from build123d import *

# Parameters (mm, degrees)
SKETCH1_R           = 3
BOSS_EXTRUDE1_DEPTH = 1.3
CHAMFER1_SIZE       = 1
SKETCH2_R           = 2
BOSS_EXTRUDE2_DEPTH = 2
CUT_EXTRUDE3_DEPTH  = 1
FILLET1_R           = 0.1
FILLET2_R           = 0.1


with BuildPart() as part:
    # Sketch1 → Boss-Extrude1 (new body)
    with BuildSketch(Plane(origin=(0, 0, 0), x_dir=(0, 0, -1), z_dir=(1, 0, 0))):
        Circle(SKETCH1_R)
    extrude(amount=BOSS_EXTRUDE1_DEPTH)

    # Chamfer1
    chamfer1_edges = [part.edges().sort_by_distance(p)[0] for p in [
        (0, 0, 3),
    ]]
    chamfer(chamfer1_edges, length=CHAMFER1_SIZE)

    # Sketch2 → Boss-Extrude2 (add)
    with BuildSketch(Plane.ZY):
        with Locations(Location((0, 0, 0), (0, 0, 180))):
            Circle(SKETCH2_R)
    extrude(amount=BOSS_EXTRUDE2_DEPTH)

    # Sketch4 → Cut-Extrude3 (cut)
    with BuildSketch(Plane(origin=(1.3, 0, 0), x_dir=(0, 0, -1), z_dir=(1, 0, 0))):
        Polygon((0.880205355, -0.907790138), (1.264303737, -0.019505387), (0.907790138, 0.880205355), (0.019505387, 1.264303737), (-0.880205355, 0.907790138), (-1.264303737, 0.019505387), (-0.907790138, -0.880205355), (-0.019505387, -1.264303737), align=None)
    extrude(amount=-CUT_EXTRUDE3_DEPTH, mode=Mode.SUBTRACT)

    # Fillet1
    fillet1_edges = [part.edges().sort_by_distance(p)[0] for p in [
        (0.3, -0.463647763, -1.072254546),
        (0.8, -0.019505387, -1.264303737),
        (0.3, -1.086046938, -0.430349984),
        (0.8, -0.907790138, -0.880205355),
        (0.3, -1.072254546, 0.463647763),
        (0.8, -1.264303737, 0.019505387),
        (0.3, -0.430349984, 1.086046938),
        (0.8, -0.880205355, 0.907790138),
        (0.3, 0.463647763, 1.072254546),
        (0.8, 0.019505387, 1.264303737),
        (0.3, 1.086046938, 0.430349984),
        (0.8, 0.907790138, 0.880205355),
        (0.3, 1.072254546, -0.463647763),
        (0.8, 1.264303737, -0.019505387),
        (0.3, 0.430349984, -1.086046938),
        (0.8, 0.880205355, -0.907790138),
        (1.3, -0.463647763, -1.072254546),
        (1.3, 0.430349984, -1.086046938),
        (1.3, 1.072254546, -0.463647763),
        (1.3, 1.086046938, 0.430349984),
        (1.3, 0.463647763, 1.072254546),
        (1.3, -0.430349984, 1.086046938),
        (1.3, -1.072254546, 0.463647763),
        (1.3, -1.086046938, -0.430349984),
    ]]
    fillet(fillet1_edges, radius=FILLET1_R)

    # Fillet2
    fillet2_edges = [part.edges().sort_by_distance(p)[0] for p in [
        (1.3, 0, 3),
        (1, 0, 3),
    ]]
    fillet(fillet2_edges, radius=FILLET2_R)


solid = part.part
For this review, take the finished solid that the model builds, in its own axes (mm). Coordinates: 2 decimals unless noted, no trailing zeros. Write each loop counter-clockwise with the first axis right and the second up, starting at its lowest first coordinate (ties: lowest second). Pieces come first, ordered by that corner, then holes. Notation, with made-up numbers: (78.5, 62.5) -> (84.5, 62.5) arc R25 ccw to (84.5, 88.5) -> close; hole circle Ø1 at (59.25, 9.5). An arc over 180 degrees is marked (long way). Write each question's results on one line, items separated by ' | '. Start each with the question number.
1) Wall thickness on L1, parallel to Z at x = 0.95, y = -0.75; L2, parallel to Z at x = 0.8, y = 0; L3, parallel to Y at x = 1, z = -0.25: over which ranges is each line inside the solid? List them lowest first. Write a range as [from, to].
2) Insertion check: pin 1 (1.5 mm diameter, centred on x = 0, y = 0.5, fed in from +Z); pin 2 (0.7 mm diameter, centred on y = -0.5, z = 0, fed in from +X); pin 3 (1 mm diameter, centred on x = 0, y = 0, fed in from -Z). Each pin has a flat end and moves straight along its axis. Give the tip position at first contact, or say it passes through.
3) The part is to be moulded in two halves that separate along Z. For faces 1 (the face through (-2, 0, 0)), 2 (the face through (-1, 2, 0)), 3 (the face through (0.3, 0, 0)), say which applies: +Z half, -Z half, draft (parallel to the pull), parting line (faces both ways), or undercut.
4) Consider section A-A (x = 0.5). Write out the cut boundary in (y, z), plus the area to 3 significant figures.
5) Consider section B-B (x = -0.5). Write out the cut boundary in (y, z), plus the area to 3 significant figures.
Geometry says:
1) L1: [-2.85, -0.95], [0.96, 2.85] | L2: [-2.8, -1.25], [1.25, 2.8] | L3: [-2.98, -1.16], [1.16, 2.98]
2) pin 1: z = 2.71 | pin 2: x = 0.3 | pin 3: z = -2.5
3) face 1: draft | face 2: parting line | face 3: undercut
4) outline: circle Ø5 at (0, 0); hole (-1.25, -0.02) -> (-0.92, -0.84) arc R0.1 ccw to (-0.87, -0.9) -> (-0.06, -1.25) arc R0.1 ccw to (0.02, -1.25) -> (0.84, -0.92) arc R0.1 ccw to (0.9, -0.87) -> (1.25, -0.06) arc R0.1 ccw to (1.25, 0.02) -> (0.92, 0.84) arc R0.1 ccw to (0.87, 0.9) -> (0.06, 1.25) arc R0.1 ccw to (-0.02, 1.25) -> (-0.84, 0.92) arc R0.1 ccw to (-0.9, 0.87) -> (-1.25, 0.06) arc R0.1 ccw to start | area: 15.1 mm^2
5) outline: circle Ø4 at (0, 0) | area: 12.6 mm^2
